Autodesk Fusion 360 part; units mm, degrees
sketch "Skizze1" plane through (0, 0, 0) normal (0, 0, 1) x (1, 0, 0)
  line L0 (-30, 35) -> (32, 35)
  line L1 (32, 35) -> (32, -45)
  line L2 (32, -45) -> (-30, -45)
  line L3 (-30, -45) -> (-30, 35)
  line L4 (34, 37) -> (34, -47)
  line L5 (34, -47) -> (-32, -47)
  line L6 (-32, -47) -> (-32, 37)
  line L7 (-32, 37) -> (34, 37)
  dimension "d1" = 62
  dimension "d2" = 80
  dimension "d3" = -2
extrude "Extrusion1" add sketch "Skizze1" along normal blind 2 contours L0 L1 L2 L3 | L4 L5 L6 L7
sketch "Skizze2" plane through (0, 0, 2) normal (0, 0, 1) x (-1, 0, 0)
  line L0 (32, -37) -> (32, 47)
  line L1 (32, 47) -> (-34, 47)
  line L2 (-34, 47) -> (-34, -37)
  line L3 (-34, -37) -> (32, -37)
  line L4 (-32, 45) -> (-32, -35)
  line L5 (-32, -35) -> (30, -35)
  line L6 (30, -35) -> (30, 45)
  line L7 (30, 45) -> (-32, 45)
  line L8 (30, -20) -> (28, -20)
  line L9 (28, -20) -> (28, 30)
  line L10 (28, 30) -> (30, 30)
  line L11 (30, 30) -> (30, -20)
  line L12 (-32, -20) -> (-30, -20)
  line L13 (-30, -20) -> (-30, 30)
  line L14 (-30, 30) -> (-32, 30)
  line L15 (-32, 30) -> (-32, -20)
  line L16 (15, 45) -> (-15, 45)
  line L17 (-15, 45) -> (-15, 43)
  line L18 (-15, 43) -> (15, 43)
  line L19 (15, 43) -> (15, 45)
  line L20 (20, -35) -> (-10, -35)
  line L21 (-10, -35) -> (-10, -33)
  line L22 (-10, -33) -> (20, -33)
  line L23 (20, -33) -> (20, -35)
  dimension "d6" = -2
  dimension "d7" = 2
  dimension "d8" = 50
  dimension "d9" = 15
  dimension "d10" = 50
  dimension "d11" = 15
  dimension "d12" = 2
  dimension "d16" = 2
  dimension "d17" = 2
  dimension "d18" = 30
  dimension "d19" = 30
  dimension "d21" = 15
  dimension "d28" = 10
extrude "Extrusion2" add sketch "Skizze2" along normal blind 4 contours L4 L12 L13 L14 L15 | L7 L16 L17 L18 L19 | L5 L20 L21 L22 L23 | L6 L8 L9 L10 L11
sketch "Skizze5" plane through (32, 0, 0) normal (1, 0, 0) x (0, 1, 0)
  line L0 (-30, 2) -> (20, 2)
  line L1 (20, 2) -> (20, 6)
  line L2 (20, 6) -> (-30, 6)
  line L3 (-30, 6) -> (-30, 2)
  line L4 (-30, 5) -> (20, 5)
  dimension "d29" = 1
extrude "Extrusion5" add sketch "Skizze5" along normal blind 0.5 contours L1 L2 L3 L4
sketch "Skizze6" plane through (-30, 0, 0) normal (-1, 0, 0) x (0, -1, 0)
  line L0 (-20, 2) -> (30, 2)
  line L1 (30, 2) -> (30, 6)
  line L2 (30, 6) -> (-20, 6)
  line L3 (-20, 6) -> (-20, 2)
  line L4 (-20, 5) -> (30, 5)
  dimension "d32" = 1
extrude "Extrusion6" add sketch "Skizze6" along normal blind 0.5 contours L1 L2 L3 L4
Can you work these out from the model? Positions are in its coordinate system, mm. A direction names the side the tool comes from. Coordinates: 2 decimals unless noted, no trailing zeros. Loops run counter-clockwise (first coordinate to the right, second up) from the corner with the lowest first, then second, coordinate; pieces in that order, holes last. Notation, with made-up numbers: M -11.5,44 L 26.5,44 A25 cw 26.5,74 Z; hole C -21,84 d11. An arc over 180 degrees is marked long. Return JSON: item names as keys, results as strings. Group by question number.
Item 1: I'm going to push flat-ended pins straight in: pin 1 Ø2 at (x, z) = (-29.5, 3.5) entering from -Y; pin 2 Ø1.5 at (y, z) = (18, 4.5) entering from +X; pin 3 Ø2 at (x, z) = (-5.5, 3.5) entering from +Y. Where does each tip first touch, or does it pass through?
Item 2: Imagine slicing it at B-B (y = -11.5). Please give me the cut outline in (x, z), and give its area (3 significant figures).
Item 3: If I drill on L1, parallel to X at y = 13, z = 3.8; L2, parallel to Y at x = 4.5, z = 2.85; L3, parallel to Z at x = 4, y = -40, over which ranges is the centre line in solid material (lowest first)? Write a range as from..to.
Item 4: Imagine slicing it at A-A (z = 3.05). Please give me the cut outline in (x, y).
Item 5: Thinking about a two-plate mould opening in Y: for faces 1 (the flat face through (-5, 33, 4)), 2 (the flat face through (-29, -30, 4)), 3 (the flat face through (31, -5, 6)), which applies, released by +Y, released by -Y, zero draft, split by the parting line, or undercut?
Item 6: On a 3-axis mill with a long thin cutter (end or side, diameter ignored), from which of +Z, -Z, +X, -X, +Y, -Y can I reach the whole of each face in a straight line? I mean faces 4 (the flat face through (-15, -44, 4)), 5 (the flat face through (-28, -5, 4)), 6 (the flat face through (-29, 20, 4)). Say none if no direction works.
Item 7: Imagine slicing it at C-C (x = -4). Please give me the cut outline in (y, z), and give its area (3 significant figures).
Item 8: Imagine slicing it at D-D (x = -22.5). Please give me the cut outline in (y, z).
Verdict:
{
 "1": {"pin 1": "stops at y = -30", "pin 2": "stops at x = 32.5", "pin 3": "stops at y = 35"},
 "2": {"outline": "M -32,0 L 34,0 L 34,2 L 32,2 L 32,5 L 32.5,5 L 32.5,6 L 30,6 L 30,2 L -28,2 L -28,6 L -30.5,6 L -30.5,5 L -30,5 L -30,2 L -32,2 Z", "area": "149 mm^2"},
 "3": {"L1": "x = -30..-28, 30..32", "L2": "y = -45..-43, 33..35", "L3": "z = 0..2"},
 "4": {"outline": "M -30,-30 L -28,-30 L -28,20 L -30,20 Z; M -20,33 L 10,33 L 10,35 L -20,35 Z; M -15,-45 L 15,-45 L 15,-43 L -15,-43 Z; M 30,-30 L 32,-30 L 32,20 L 30,20 Z"},
 "5": {"face 1": "undercut", "face 2": "released by -Y", "face 3": "zero draft"},
 "6": {"face 4": "+Z, -X, -Y", "face 5": "+Z, +Y, -Y", "face 6": "+Z, +X, -X, +Y"},
 "7": {"outline": "M -47,0 L 37,0 L 37,2 L 35,2 L 35,6 L 33,6 L 33,2 L -43,2 L -43,6 L -45,6 L -45,2 L -47,2 Z", "area": "184 mm^2"},
 "8": {"outline": "M -47,0 L 37,0 L 37,2 L -47,2 Z"}
}
